Check sheet for the modelled part. Datum: model origin and axes. Units: mm. Face numbers are marked on the shaded views. A direction names the side the tool comes from. Round coordinates to 2 decimals unless told otherwise and drop trailing zeros. Loops run counter-clockwise (first coordinate to the right, second up) from the corner with the lowest first, then second, coordinate; pieces in that order, holes last. Notation, with made-up numbers: M -23,-30.5 L 29,-30.5 A12 ccw 29,-12.5 Z; hole C -11.5,71 d4. An arc over 180 degrees is marked long. One line per question, with ' | ' between items. Start each with the question number.
(1) Section check B-B (x = -18.5). Record the boundary of the cut face in (y, z), and give its area (3 significant figures).
(2) Section check C-C (y = 0). Record the boundary of the cut face in (x, z) (3 decimals), and give its area (3 significant figures).
(3) Go/stop test with a flat-tipped pin: P1, Ø8, axis at x = 4, y = 10, coming from the -Z side. Record where the tip stops, or that it passes through.
(4) Section check D-D (x = 0). Record the boundary of the cut face in (y, z) (3 decimals).
(5) Tool access check on the marked faces 1 and 2. Record the directions out of +Z, -Z, +X, -X, +Y, -Y that give a thin tool (end or side, any length) a straight path to the whole face; none if there is none.
(6) Thickness scan on probe 1 along Y at (x, z) = (-18.5, -0.05); probe 2 along X at (y, z) = (3.75, 0.25); probe 3 along Y at (x, z) = (0, 0.25) (3 decimals). Record the ranges inside material, lowest first. Write a range as [from, to].
(7) Draft check along Y on the marked faces 3, 4 and 5. Enter one of: +Y half, -Y half, draft (parallel to the pull), parting line (faces both ways), or undercut.
(8) Section check A-A (z = 0.25). Record the boundary of the cut face in (x, y) (3 decimals).
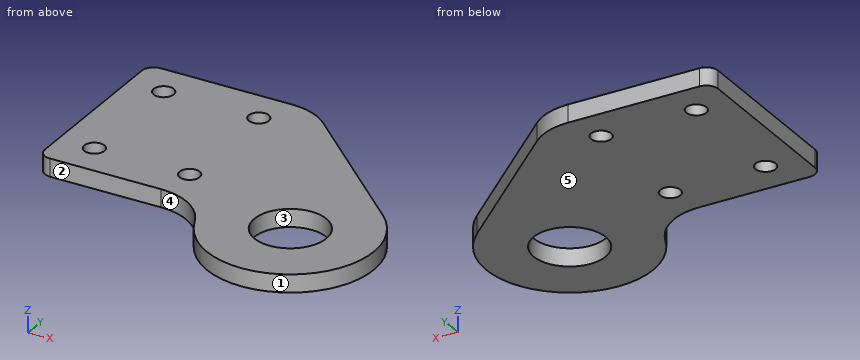
```python
from build123d import *

# Parameters (mm, degrees)
ESQUISSE1_R        = 3.025
ESQUISSE1_R_2      = 0.85
BOSS_EXTRU_1_DEPTH = 0.75
CONG_1_R           = 5
CONG_2_R           = 1


with BuildPart() as part:
    # Esquisse1 → Boss.-Extru.1 (new body, symmetric)
    with BuildSketch(Plane.XY):
        with BuildLine():
            Line((-7.5, 16.5), (4.768672746, 5.158525491))
            ThreePointArc((4.768672746, 5.158525491), (2.584220944, -6.532413575), (-7.007183814, 0.5))
            Line((-7.007183814, 0.5), (-7.5, 0.5))
            Line((-7.5, 0.5), (-21.5, 0.5))
            Line((-21.5, 0.5), (-21.5, 16.5))
            Line((-21.5, 16.5), (-7.5, 16.5))
        make_face()
        Circle(ESQUISSE1_R, mode=Mode.SUBTRACT)
        with Locations((-18.5, 13.5)):
            Circle(ESQUISSE1_R_2, mode=Mode.SUBTRACT)
        with Locations((-10.5, 13.5)):
            Circle(ESQUISSE1_R_2, mode=Mode.SUBTRACT)
        with Locations((-10.5, 3.5)):
            Circle(ESQUISSE1_R_2, mode=Mode.SUBTRACT)
        with Locations((-18.5, 3.5)):
            Circle(ESQUISSE1_R_2, mode=Mode.SUBTRACT)
    extrude(amount=BOSS_EXTRU_1_DEPTH, both=True)

    # Congé1
    cong_1_edges = [part.edges().sort_by_distance(p)[0] for p in [
        (-7.5, 16.5, 0),
        (-7.007183814, 0.5, 0),
    ]]
    fillet(cong_1_edges, radius=CONG_1_R)

    # Congé2
    cong_2_edges = [part.edges().sort_by_distance(p)[0] for p in [
        (-21.5, 16.5, 0),
        (-21.5, 0.5, 0),
    ]]
    fillet(cong_2_edges, radius=CONG_2_R)


solid = part.part
```
The answers:
1) outline: M 0.5,-0.75 L 2.65,-0.75 L 2.65,0.75 L 0.5,0.75 Z; M 4.35,-0.75 L 12.65,-0.75 L 12.65,0.75 L 4.35,0.75 Z; M 14.35,-0.75 L 16.5,-0.75 L 16.5,0.75 L 14.35,0.75 Z | area: 18.9 mm²
2) outline: M -8.972,-0.75 L -3.025,-0.75 L -3.025,0.75 L -8.972,0.75 Z; M 3.025,-0.75 L 7.025,-0.75 L 7.025,0.75 L 3.025,0.75 Z | area: 14.9 mm²
3) P1: z = -0.75
4) outline: M -7.025,-0.75 L -3.025,-0.75 L -3.025,0.75 L -7.025,0.75 Z; M 3.025,-0.75 L 9.567,-0.75 L 9.567,0.75 L 3.025,0.75 Z
5) face 1: +Z, -Z | face 2: +Z, -Z, -X, -Y
6) probe 1: [0.5, 2.65], [4.35, 12.65], [14.35, 16.5] | probe 2: [-21.5, -19.31], [-17.69, -11.31], [-9.69, 5.94] | probe 3: [-7.025, -3.025], [3.025, 9.567]
7) face 3: undercut | face 4: -Y half | face 5: draft
8) outline: M -21.5,1.5 A1 ccw -20.5,0.5 L -11.151,0.5 A5 cw -6.515,-2.629 A7.025 ccw long 4.769,5.159 L -6.063,15.172 A5 ccw -9.457,16.5 L -20.5,16.5 A1 ccw -21.5,15.5 Z; hole C -18.5,3.5 d1.7; hole C -18.5,13.5 d1.7; hole C -10.5,3.5 d1.7; hole C -10.5,13.5 d1.7; hole C 0,0 d6.05
